Can you work these out from the model? Positions are in its coordinate system, mm. A direction names the side the tool comes from. Give positions to 0.01 mm unless a question says otherwise; leave off trailing zeros. Loops run counter-clockwise (first coordinate to the right, second up) from the corner with the lowest first, then second, coordinate; pieces in that order, holes last. Notation, with made-up numbers: (28, -5) -> (41, -5) arc R25 cw to (41, 8) -> close; hole circle Ø5 at (16, 6.25). An arc over 180 degrees is marked (long way). Return JSON: item names as keys, results as strings. Group by question number.
Q1. Suppose I cut it at A-A, the plane y = 6. Please give me the cut outline in (x, z).
Q2. Will these pins go through, and if not, where does the flat tip stop? pin 1 (3 mm diameter, centred on y = 11.5, z = 2, fed in from -X); pin 2 (1.7 mm diameter, centred on y = -14, z = 1.5, fed in from +X); pin 3 (1.5 mm diameter, centred on y = -23, z = 1, fed in from +X).
Q3. Suppose I cut it at B-B, the plane x = 28.5. Please give me the cut outline in (y, z).
Q4. Which directions (+Z, -Z, +X, -X, +Y, -Y) give clear straight access to the entire face, cutting with the end or side of a thin tool? Please do faces 3 (the flat face through (-0.604, -13.036, 2.465)), 4 (the flat face through (-6.5, -9.2, 5)).
Q5. Suppose I cut it at D-D, the plane z = 1.8. Count the separate pieces of the cut face and the enclosed holes in it, and give its area (3 significant figures).
Q6. Suppose I cut it at C-C, the plane y = -3.5. Please give me the cut outline in (x, z).
Q7. I need wall thicknesses on line 1 along Y through (x, z) = (2.5, 3.85); line 2 along Y through (x, z) = (-9.5, 4.6); line 3 along X through (y, z) = (1, 0.8). Which ranges of each line are inside material? Lowest first, please. Write a range as [from, to].
Q8. Thinking about a two-plate mould opening in X: for faces 1 (the flat face through (-6.5, -9.2, 0)), 2 (the flat face through (1.636, -13, 2)), which applies, pulls with the +X half, pulls with the -X half, needs draft (parallel to the pull), parting line crosses it, or undercut?
```python
from build123d import *

# Parameters (mm, degrees)
F0_R     = 11
F1_DEPTH = 5


with BuildPart() as f1:
    # F0 (on Top) → F1 (new body)
    with BuildSketch(Plane.XY):
        with BuildLine():
            ThreePointArc((24.3693606457, 12.0805580484), (24.0077279335, 11.9071162023), (23.6389782963, 11.7493695776))
            ThreePointArc((23.6389782963, 11.7493695776), (16.3793921161, 0.5682163901), (22.7809509477, -11.1253640126))
            ThreePointArc((22.7809509477, -11.1253640126), (24.1883269703, -11.6184397697), (25.4992191241, -12.3293495618))
            ThreePointArc((25.4992191241, -12.3293495618), (37.0733893442, -10.3910189502), (42.3702563381, 0.0809312927))
            ThreePointArc((42.3702563381, 0.0809312927), (36.5809551946, 10.8978542378), (24.3693606457, 12.0805580484))
        make_face()
        with Locations((29.3702563381, 0.0809312927)):
            Circle(F0_R, mode=Mode.SUBTRACT)
        with BuildLine():
            ThreePointArc((12.0805580484, -24.3693606457), (11.9071162023, -24.0077279335), (11.7493695776, -23.6389782963))
            ThreePointArc((11.7493695776, -23.6389782963), (0.5682163901, -16.3793921161), (-11.1253640126, -22.7809509477))
            ThreePointArc((-11.1253640126, -22.7809509477), (-11.6184397697, -24.1883269703), (-12.3293495618, -25.4992191241))
            ThreePointArc((-12.3293495618, -25.4992191241), (-1.8769181513, -42.2219809521), (13.0809312927, -29.3702563381))
            ThreePointArc((13.0809312927, -29.3702563381), (12.8283849173, -26.8202708306), (12.0805580484, -24.3693606457))
        make_face()
        with Locations((0.0809312927, -29.3702563381)):
            Circle(F0_R, mode=Mode.SUBTRACT)
        with BuildLine():
            ThreePointArc((-16.3702563381, -0.0809312927), (-18.0861752928, 6.3742615752), (-22.7809509477, 11.1253640126))
            ThreePointArc((-22.7809509477, 11.1253640126), (-24.1883269703, 11.6184397697), (-25.4992191241, 12.3293495618))
            ThreePointArc((-25.4992191241, 12.3293495618), (-42.3563525859, -0.6820171789), (-24.3693606457, -12.0805580484))
            ThreePointArc((-24.3693606457, -12.0805580484), (-24.0077279335, -11.9071162023), (-23.6389782963, -11.7493695776))
            ThreePointArc((-23.6389782963, -11.7493695776), (-18.336068227, -6.9545542624), (-16.3702563381, -0.0809312927))
        make_face()
        with Locations((-29.3702563381, -0.0809312927)):
            Circle(F0_R, mode=Mode.SUBTRACT)
        with BuildLine():
            ThreePointArc((12.3293495618, 25.4992191241), (12.7707933213, 27.412406894), (12.9190687073, 29.3702563381))
            ThreePointArc((12.9190687073, 29.3702563381), (-2.6309168002, 42.1177099627), (-12.0805580484, 24.3693606457))
            ThreePointArc((-12.0805580484, 24.3693606457), (-11.9071162023, 24.0077279335), (-11.7493695776, 23.6389782963))
            ThreePointArc((-11.7493695776, 23.6389782963), (-0.5682163901, 16.3793921161), (11.1253640126, 22.7809509477))
            ThreePointArc((11.1253640126, 22.7809509477), (11.6184397697, 24.1883269703), (12.3293495618, 25.4992191241))
        make_face()
        with Locations((-0.0809312927, 29.3702563381)):
            Circle(F0_R, mode=Mode.SUBTRACT)
        with BuildLine():
            ThreePointArc((11.1253640126, 22.7809509477), (-0.5682163901, 16.3793921161), (-11.7493695776, 23.6389782963))
            ThreePointArc((-11.7493695776, 23.6389782963), (-13.4063117417, 13.9803401177), (-22.7809509477, 11.1253640126))
            ThreePointArc((-22.7809509477, 11.1253640126), (-18.0861752928, 6.3742615752), (-16.3702563381, -0.0809312927))
            ThreePointArc((-16.3702563381, -0.0809312927), (-18.336068227, -6.9545542624), (-23.6389782963, -11.7493695776))
            ThreePointArc((-23.6389782963, -11.7493695776), (-13.9803401177, -13.4063117417), (-11.1253640126, -22.7809509477))
            ThreePointArc((-11.1253640126, -22.7809509477), (0.5682163901, -16.3793921161), (11.7493695776, -23.6389782963))
            ThreePointArc((11.7493695776, -23.6389782963), (13.4063117417, -13.9803401177), (22.7809509477, -11.1253640126))
            ThreePointArc((22.7809509477, -11.1253640126), (16.3793921161, 0.5682163901), (23.6389782963, 11.7493695776))
            ThreePointArc((23.6389782963, 11.7493695776), (13.9803401177, 13.4063117417), (11.1253640126, 22.7809509477))
        make_face()
        Polygon((-6.780023326, -14.6987217482), (-6.780023326, -15.0520168245), (-8.6744287142, -15.0520168245), (-8.6744287142, -11.6536900799), (-6.780023326, -11.6536900799), (-6.780023326, -12.0047538189), (-8.2794820078, -12.0047538189), (-8.2794820078, -13.0995966659), (-6.8707643772, -13.0995966659), (-6.8707643772, -13.4484290676), (-8.2794820078, -13.4484290676), (-8.2794820078, -14.6987217482), align=None, mode=Mode.SUBTRACT)
        with BuildLine():
            Line((-4.205060054, -15.0520168245), (-4.5233975123, -15.0520168245))
            Line((-4.5233975123, -15.0520168245), (-5.6762551297, -12.039711437))
            Line((-5.6762551297, -12.039711437), (-5.6948496074, -12.039711437))
            add(Edge.make_bspline(
                [(-5.6948496074, -12.039711437), (-5.6621233267, -12.3974691879), (-5.6621233267, -12.8905947365)],
                knots=[0, 0, 0, 1, 1, 1], degree=2))
            Line((-5.6621233267, -12.8905947365), (-5.6621233267, -15.0520168245))
            Line((-5.6621233267, -15.0520168245), (-6.0273188687, -15.0520168245))
            Line((-6.0273188687, -15.0520168245), (-6.0273188687, -11.6536900799))
            Line((-6.0273188687, -11.6536900799), (-5.4322955823, -11.6536900799))
            Line((-5.4322955823, -11.6536900799), (-4.3560472129, -14.4569935381))
            Line((-4.3560472129, -14.4569935381), (-4.3374527352, -14.4569935381))
            Line((-4.3374527352, -14.4569935381), (-3.2522790166, -11.6536900799))
            Line((-3.2522790166, -11.6536900799), (-2.6617184049, -11.6536900799))
            Line((-2.6617184049, -11.6536900799), (-2.6617184049, -15.0520168245))
            Line((-2.6617184049, -15.0520168245), (-3.0566651112, -15.0520168245))
            Line((-3.0566651112, -15.0520168245), (-3.0566651112, -12.8623311304))
            add(Edge.make_bspline(
                [(-3.0566651112, -12.8623311304), (-3.0566651112, -12.4859789018), (-3.0239388305, -12.0441741116)],
                knots=[0, 0, 0, 1, 1, 1], degree=2))
            Line((-3.0239388305, -12.0441741116), (-3.0425333082, -12.0441741116))
            Line((-3.0425333082, -12.0441741116), (-4.205060054, -15.0520168245))
        make_face(mode=Mode.SUBTRACT)
        with BuildLine():
            Line((0.0924956322, -15.0520168245), (-0.225841826, -15.0520168245))
            Line((-0.225841826, -15.0520168245), (-1.3786994435, -12.039711437))
            Line((-1.3786994435, -12.039711437), (-1.3972939212, -12.039711437))
            add(Edge.make_bspline(
                [(-1.3972939212, -12.039711437), (-1.3645676404, -12.3974691879), (-1.3645676404, -12.8905947365)],
                knots=[0, 0, 0, 1, 1, 1], degree=2))
            Line((-1.3645676404, -12.8905947365), (-1.3645676404, -15.0520168245))
            Line((-1.3645676404, -15.0520168245), (-1.7297631825, -15.0520168245))
            Line((-1.7297631825, -15.0520168245), (-1.7297631825, -11.6536900799))
            Line((-1.7297631825, -11.6536900799), (-1.1347398961, -11.6536900799))
            Line((-1.1347398961, -11.6536900799), (-0.0584915267, -14.4569935381))
            Line((-0.0584915267, -14.4569935381), (-0.039897049, -14.4569935381))
            Line((-0.039897049, -14.4569935381), (1.0452766696, -11.6536900799))
            Line((1.0452766696, -11.6536900799), (1.6358372814, -11.6536900799))
            Line((1.6358372814, -11.6536900799), (1.6358372814, -15.0520168245))
            Line((1.6358372814, -15.0520168245), (1.240890575, -15.0520168245))
            Line((1.240890575, -15.0520168245), (1.240890575, -12.8623311304))
            add(Edge.make_bspline(
                [(1.240890575, -12.8623311304), (1.240890575, -12.4859789018), (1.2736168557, -12.0441741116)],
                knots=[0, 0, 0, 1, 1, 1], degree=2))
            Line((1.2736168557, -12.0441741116), (1.255022378, -12.0441741116))
            Line((1.255022378, -12.0441741116), (0.0924956322, -15.0520168245))
        make_face(mode=Mode.SUBTRACT)
        Polygon((4.4621978919, -14.6987217482), (4.4621978919, -15.0520168245), (2.5677925037, -15.0520168245), (2.5677925037, -11.6536900799), (4.4621978919, -11.6536900799), (4.4621978919, -12.0047538189), (2.9627392101, -12.0047538189), (2.9627392101, -13.0995966659), (4.3714568407, -13.0995966659), (4.3714568407, -13.4484290676), (2.9627392101, -13.4484290676), (2.9627392101, -14.6987217482), align=None, mode=Mode.SUBTRACT)
        Polygon((6.2606557751, -12.0047538189), (6.2606557751, -15.0520168245), (5.8657090687, -15.0520168245), (5.8657090687, -12.0047538189), (4.7894606994, -12.0047538189), (4.7894606994, -11.6536900799), (7.3369041444, -11.6536900799), (7.3369041444, -12.0047538189), align=None, mode=Mode.SUBTRACT)
        Polygon((8.8943775966, -12.0047538189), (8.8943775966, -15.0520168245), (8.4994308903, -15.0520168245), (8.4994308903, -12.0047538189), (7.423182521, -12.0047538189), (7.423182521, -11.6536900799), (9.970625966, -11.6536900799), (9.970625966, -12.0047538189), align=None, mode=Mode.SUBTRACT)
        Circle(F0_R, mode=Mode.SUBTRACT)
    extrude(amount=F1_DEPTH)


solid = f1.part
```
Ans:
{
 "1": {"outline": "(-40.86, 0) -> (-38.54, 0) -> (-38.54, 5) -> (-40.86, 5) -> close; (-20.2, 0) -> (-9.22, 0) -> (-9.22, 5) -> (-20.2, 5) -> close; (9.22, 0) -> (20.1, 0) -> (20.1, 5) -> (9.22, 5) -> close; (38.64, 0) -> (40.94, 0) -> (40.94, 5) -> (38.64, 5) -> close"},
 "2": {"pin 1": "stops at x = -37.58", "pin 2": "stops at x = 14.24", "pin 3": "stops at x = 11.79"},
 "3": {"outline": "(-12.89, 0) -> (-10.88, 0) -> (-10.88, 5) -> (-12.89, 5) -> close; (11.05, 0) -> (13.05, 0) -> (13.05, 5) -> (11.05, 5) -> close"},
 "4": {"face 3": "+Z, -Z", "face 4": "+Z, +X, -X, +Y, -Y"},
 "5": {"separate pieces": "1", "enclosed holes": "11", "area": "1,390 mm^2"},
 "6": {"outline": "(-41.91, 0) -> (-39.83, 0) -> (-39.83, 5) -> (-41.91, 5) -> close; (-18.92, 0) -> (-10.43, 0) -> (-10.43, 5) -> (-18.92, 5) -> close; (10.43, 0) -> (18.97, 0) -> (18.97, 5) -> (10.43, 5) -> close; (39.77, 0) -> (41.87, 0) -> (41.87, 5) -> (39.77, 5) -> close"},
 "7": {"line 1": "y = [-42.14, -40.1], [-18.64, -10.71], [10.71, 18.68], [40.06, 42.11]", "line 2": "y = [-38.16, -34.77], [-23.97, -5.55], [5.55, 23.69], [35.05, 38.33]", "line 3": "x = [-42.33, -40.32], [-18.42, -10.95], [10.95, 18.41], [40.33, 42.34]"},
 "8": {"face 1": "needs draft", "face 2": "undercut"}
}
